Geometry: final body of the model. Coordinates: model frame, mm. A direction names the side the tool comes from. Coordinates: 2 decimals unless noted, no trailing zeros. Write each loop counter-clockwise with the first axis right and the second up, starting at its lowest first coordinate (ties: lowest second). Pieces come first, ordered by that corner, then holes.
from build123d import *

# Parameters (mm, degrees)
SKETCH1_R           = 2.3
BOSS_EXTRUDE1_DEPTH = 1
SKETCH2_R           = 1.75
SKETCH2_R_2         = 1
BOSS_EXTRUDE2_DEPTH = 5
BOSS_EXTRUDE3_DEPTH = 5
CIRPATTERN1_COUNT   = 8


with BuildPart() as part:
    # Sketch1 → Boss-Extrude1 (new body)
    with BuildSketch(Plane(origin=(0, 0, 0), x_dir=(0, 0, -1), z_dir=(1, 0, 0))):
        Circle(SKETCH1_R)
    extrude(amount=BOSS_EXTRUDE1_DEPTH)

    # Sketch2 → Boss-Extrude2 (add)
    with BuildSketch(Plane(origin=(1, 0, 0), x_dir=(0, 0, -1), z_dir=(1, 0, 0))):
        Circle(SKETCH2_R)
        Circle(SKETCH2_R_2, mode=Mode.SUBTRACT)
    extrude(amount=BOSS_EXTRUDE2_DEPTH)


with BuildPart() as body_2:
    # Sketch3 → Boss-Extrude3 (new body)
    with BuildSketch(Plane(origin=(1, 0, 0), x_dir=(0, 0, -1), z_dir=(1, 0, 0))):
        with BuildLine():
            ThreePointArc((-0.45982072, 1.68850967), (0, 1.75), (0.45982072, 1.68850967))
            Line((0.45982072, 1.68850967), (0.45982072, 2.253567151))
            ThreePointArc((0.45982072, 2.253567151), (0.359046611, 2.672132166), (0.078809895, 2.998964655))
            ThreePointArc((0.078809895, 2.998964655), (0, 3), (-0.078809895, 2.998964655))
            ThreePointArc((-0.078809895, 2.998964655), (-0.359046611, 2.672132166), (-0.45982072, 2.253567151))
            Line((-0.45982072, 2.253567151), (-0.45982072, 1.68850967))
        make_face()
    extrude(amount=BOSS_EXTRUDE3_DEPTH)


with BuildPart() as cirpattern1_1:
    # CirPattern1: pattern copy
    add(body_2.part.rotate(Axis((0, 0, 0), (1, 0, 0)), 1 * 360 / CIRPATTERN1_COUNT))


with BuildPart() as cirpattern1_2:
    # CirPattern1: pattern copy
    add(body_2.part.rotate(Axis((0, 0, 0), (1, 0, 0)), 2 * 360 / CIRPATTERN1_COUNT))


with BuildPart() as cirpattern1_3:
    # CirPattern1: pattern copy
    add(body_2.part.rotate(Axis((0, 0, 0), (1, 0, 0)), 3 * 360 / CIRPATTERN1_COUNT))


with BuildPart() as cirpattern1_4:
    # CirPattern1: pattern copy
    add(body_2.part.rotate(Axis((0, 0, 0), (1, 0, 0)), 4 * 360 / CIRPATTERN1_COUNT))


with BuildPart() as cirpattern1_5:
    # CirPattern1: pattern copy
    add(body_2.part.rotate(Axis((0, 0, 0), (1, 0, 0)), 5 * 360 / CIRPATTERN1_COUNT))


with BuildPart() as cirpattern1_6:
    # CirPattern1: pattern copy
    add(body_2.part.rotate(Axis((0, 0, 0), (1, 0, 0)), 6 * 360 / CIRPATTERN1_COUNT))


with BuildPart() as cirpattern1_7:
    # CirPattern1: pattern copy
    add(body_2.part.rotate(Axis((0, 0, 0), (1, 0, 0)), 7 * 360 / CIRPATTERN1_COUNT))


with BuildPart() as body_2_1:
    add(body_2.part)

    # Combine1: union CirPattern1_7, CirPattern1_6, CirPattern1_4, CirPattern1_3, part, CirPattern1_1, CirPattern1_2, CirPattern1_5
    add(cirpattern1_7.part)
    add(cirpattern1_6.part)
    add(cirpattern1_4.part)
    add(cirpattern1_3.part)
    add(part.part)
    add(cirpattern1_1.part)
    add(cirpattern1_2.part)
    add(cirpattern1_5.part)


solid = body_2_1.part
Item 1: Pin query (flat end, axial travel): pin 1 (2 mm diameter, centred on x = 3, y = -2, fed in from +Z); pin 2 (1.5 mm diameter, centred on x = 1.5, y = 1, fed in from +Z); pin 3 (0.5 mm diameter, centred on x = 2.5, z = 2, fed in from -Y). Return the tip coordinate at first contact, or that it passes through.
Derived:
pin 1: stops at z = 2.19
pin 2: stops at z = 2.84
pin 3: stops at y = -2.19
Item 2: Set-up query: faces 1 (the flat face through (1, 0, 0)), 2 (the flat face through (1, 2, -2)), 3 (the flat face through (1, -2, -2)), 4 (the flat face through (0, 0, 0)), 5 (the flat face through (1, 2, 2)). Return all of +Z, -Z, +X, -X, +Y, -Y with unobstructed straight access to the full face (end or side cutting, diameter ignored); none if empty.
Derived:
face 1: +X
face 2: -Z, -X, +Y
face 3: -Z, -X, -Y
face 4: +Z, -Z, -X, +Y, -Y
face 5: +Z, -X, +Y
Item 3: Pull-direction query (Z, two-part tool) for faces 6 (the flat face through (1, -2, 2)), 7 (the cylindrical face through (3, -1, 0)), 8 (the cylindrical face through (0.493, -1.4, 1.825)); classes: released by +Z, released by -Z, zero draft, split by the parting line, or undercut.
Derived:
face 6: zero draft
face 7: undercut
face 8: split by the parting line
Item 4: Section A-A, the plane y = -1.1. Output: boundary loops of the cut face in (x, z).
Derived:
outline: (0, -2.02) - (1, -2.02) - (1, -1.75) - (6, -1.75) - (6, 1.75) - (1, 1.75) - (1, 2.02) - (0, 2.02) - close
Item 5: Material intervals for probe 1 along Y at (x, z) = (2.5, 0); probe 2 along Z at (x, y) = (3.45, -1.6); probe 3 along Z at (x, y) = (3.95, -2.05), sorted ascending.
Derived:
probe 1: y = -3 to -1, 1 to 3
probe 2: z = -2.13 to -0.95, -0.71 to 0.71, 0.95 to 2.13
probe 3: z = -2.18 to -1.43, -0.46 to 0.46, 1.43 to 2.18
Item 6: Section B-B, the plane y = 2.5. Output: boundary loops of the cut face in (x, z).
Derived:
outline: (1, -0.43) - (6, -0.43) - (6, 0.43) - (1, 0.43) - close
